Build history of the part. All positions in model axes, mm. Face numbers are marked on the shaded views. Give positions to 0.01 mm unless a question says otherwise; leave off trailing zeros. Write each loop counter-clockwise with the first axis right and the second up, starting at its lowest first coordinate (ties: lowest second). Pieces come first, ordered by that corner, then holes. Notation, with made-up numbers: (36.25, 26) -> (56.25, 26) arc R30 ccw to (56.25, 54) -> close; hole circle Ø1 at (-17.5, 57.5). An arc over 180 degrees is marked (long way). Put each result on its own line as item: value. Start each with the question number.
Item 1: Slice it at D-D, the plane x = 0. List the corners of the cut face in (y, z).
Item 2: Slice it at B-B, the plane x = -2.5. List the corners of the cut face in (y, z), plus the area to 3 significant figures.
Item 3: Slice it at A-A, the plane z = -2.5. List the corners of the cut face in (x, y).
Item 4: Two-plate mould, pull along Y, no slides. Class the marked faces 1, 2 and 3: pulls with the +Y half, pulls with the -Y half, needs draft (parallel to the pull), parting line crosses it, or undercut.
Item 5: Drill centre lines: line 1 along Y through (x, z) = (0.25, 3.75); line 2 along X through (y, z) = (13, 0); line 3 along Z through (x, y) = (1.75, 9.5). Where is each one in solid material? Low to high.
Item 6: Slice it at C-C, the plane z = 0. List the corners of the cut face in (x, y), plus the area to 3 significant figures.
Item 7: Flat gauge pins, fed straight in: pin 1 Ø1.5 at (y, z) = (5, -0.5) entering from +X; pin 2 Ø3 at (y, z) = (9.5, -2) entering from +X (3 decimals); pin 3 Ø2 at (x, y) = (1.5, 2.5) entering from -Z (3 decimals). Where does each tip first touch, or does it go through?
```python
from build123d import *

# Parameters (mm, degrees)
SKETCH1_R           = 2.3
BOSS_EXTRUDE1_DEPTH = 18.2
BOSS_EXTRUDE2_START = 9.1
SKETCH2_R           = 4
SKETCH2_R_2         = 2.3
BOSS_EXTRUDE2_DEPTH = 1
BOSS_EXTRUDE3_START = -9.1
SKETCH2_3_R         = 4
SKETCH2_3_R_2       = 2.3
BOSS_EXTRUDE3_DEPTH = 1


with BuildPart() as part:
    # Sketch1 → Boss-Extrude1 (new body)
    with BuildSketch(Plane(origin=(0, 0, 0), x_dir=(1, 0, 0), z_dir=(0, 1, 0))):
        Circle(SKETCH1_R)
    extrude(amount=BOSS_EXTRUDE1_DEPTH)

    # Sketch2 → Boss-Extrude2 (add)
    with BuildSketch(Plane(origin=(0, 9.1, 0), x_dir=(1, 0, 0), z_dir=(0, 1, 0)).offset(BOSS_EXTRUDE2_START)):
        Circle(SKETCH2_R)
        Circle(SKETCH2_R_2, mode=Mode.SUBTRACT)
    extrude(amount=-BOSS_EXTRUDE2_DEPTH)

    # Sketch2<3> → Boss-Extrude3 (add)
    with BuildSketch(Plane(origin=(0, 9.1, 0), x_dir=(1, 0, 0), z_dir=(0, 1, 0)).offset(BOSS_EXTRUDE3_START)):
        Circle(SKETCH2_3_R)
        Circle(SKETCH2_3_R_2, mode=Mode.SUBTRACT)
    extrude(amount=BOSS_EXTRUDE3_DEPTH)


solid = part.part
```
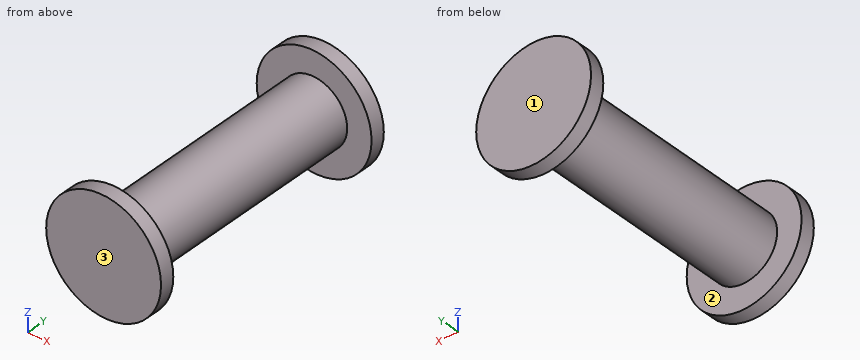
Values follow:
1. outline: (0, -4) -> (1, -4) -> (1, -2.3) -> (17.2, -2.3) -> (17.2, -4) -> (18.2, -4) -> (18.2, 4) -> (17.2, 4) -> (17.2, 2.3) -> (1, 2.3) -> (1, 4) -> (0, 4) -> close
2. outline: (0, -3.12) -> (1, -3.12) -> (1, 3.12) -> (0, 3.12) -> close; (17.2, -3.12) -> (18.2, -3.12) -> (18.2, 3.12) -> (17.2, 3.12) -> close
2. area: 12.5 mm2
3. outline: (-3.12, 0) -> (3.12, 0) -> (3.12, 1) -> (-3.12, 1) -> close; (-3.12, 17.2) -> (3.12, 17.2) -> (3.12, 18.2) -> (-3.12, 18.2) -> close
4. face 1: pulls with the +Y half
4. face 2: undercut
4. face 3: pulls with the -Y half
5. line 1: 0 to 1, 17.2 to 18.2
5. line 2: -2.3 to 2.3
5. line 3: -1.49 to 1.49
6. outline: (-4, 0) -> (4, 0) -> (4, 1) -> (2.3, 1) -> (2.3, 17.2) -> (4, 17.2) -> (4, 18.2) -> (-4, 18.2) -> (-4, 17.2) -> (-2.3, 17.2) -> (-2.3, 1) -> (-4, 1) -> close
6. area: 90.5 mm2
7. pin 1: x = 2.3
7. pin 2: x = 2.245
7. pin 3: z = -2.245
